Autodesk Inventor part; units mm, degrees
ref_plane "YZ Plane" through (0, 0, 0) normal (1, 0, 0) x (0, 1, 0)
ref_plane "XZ Plane" through (0, 0, 0) normal (0, 1, 0) x (-1, 0, 0)
ref_plane "XY Plane" through (0, 0, 0) normal (0, 0, 1) x (1, 0, 0)
sketch "Sketch1" plane through (0, 0, 0) normal (0, 1, 0) x (-1, 0, 0)
  line L0 (-17.5, 16.9) -> (17.5, 16.9)
  line L1 (17.5, 16.9) -> (17.5, -16.9)
  line L2 (17.5, -16.9) -> (-17.5, -16.9)
  line L3 (-17.5, -16.9) -> (-17.5, 16.9)
  line L4 (-17.5, 16.9) -> (17.5, -16.9) construction
  line L5 (17.5, 16.9) -> (-17.5, -16.9) construction
  point P0 (0, 0)
sketch "Sketch2" plane through (0, 0, 0) normal (0, 1, 0) x (-1, 0, 0)
  line L0 (980.2308, 0) -> (977.7308, 0)
  line L1 (17.4632, -0.049) -> (15.105, -0.049)
  line L2 (12.1095, 2.9465) -> (18.1005, 2.9465)
  line L3 (18.1005, 2.9465) -> (18.1005, -3.0446)
  line L4 (18.1005, -3.0446) -> (12.1095, -3.0446)
  line L5 (12.1095, -3.0446) -> (12.1095, 2.9465)
  line L6 (12.1095, 2.9465) -> (18.1005, -3.0446) construction
  line L7 (18.1005, 2.9465) -> (12.1095, -3.0446) construction
  line L8 (12.4632, 12.2678) -> (18.1005, 12.2678)
  line L9 (18.1005, 12.2678) -> (18.1005, 6.638)
  line L10 (18.1005, 6.638) -> (12.4632, 6.638)
  line L11 (12.4632, 6.638) -> (12.4632, 12.2678)
  line L12 (12.4632, 12.2678) -> (18.1005, 6.638) construction
  line L13 (12.0658, -6.5864) -> (18.1005, -6.5864)
  line L14 (18.1005, -6.5864) -> (18.1005, -12.7382)
  line L15 (18.1005, -12.7382) -> (12.0658, -12.7382)
  line L16 (12.0658, -12.7382) -> (12.0658, -6.5864)
  line L17 (12.0658, -6.5864) -> (18.1005, -12.7382) construction
  line L18 (18.1005, -6.5864) -> (12.0658, -12.7382) construction
  point P0 (0, 0)
  dimension "d2" = 2.5
extrude "Extrusion1" add sketch "Sketch1" along normal blind 4
extrude "Extrusion2" cut sketch "Sketch2" along normal blind 4
fillet "Fillet3" radius 2 1 edges at (17.5, 4, 0)
fillet "Fillet4" radius 2 1 edges at (17.5, 0, 0)
sketch "Sketch3" plane through (0, 4, 0) normal (0, 1, 0) x (1, 0, 0)
  line L0 (-17.5, 3.0446) -> (-12.1095, 3.0446) construction
  line L1 (-12.1095, 3.0446) -> (-12.1095, -2.9465) construction
  line L2 (-12.1095, -2.9465) -> (-17.5, -2.9465) construction
  line L3 (-17.5, -2.9465) -> (-17.5, -6.638) construction
  line L4 (-17.5, -6.638) -> (-12.4632, -6.638) construction
  line L5 (-12.4632, -6.638) -> (-12.4632, -12.2678) construction
  line L6 (-12.4632, -12.2678) -> (-17.5, -12.2678) construction
  line L7 (-17.5, -12.2678) -> (-17.5, -16.9) construction
  line L8 (-17.5, -16.9) -> (15.5, -16.9) construction
  line L9 (15.5, 16.9) -> (-17.5, 16.9) construction
  line L10 (-17.5, 16.9) -> (-17.5, 12.7382) construction
  line L11 (-17.5, 12.7382) -> (-12.0658, 12.7382) construction
  line L12 (-12.0658, 12.7382) -> (-12.0658, 6.5864) construction
  line L13 (-12.0658, 6.5864) -> (-17.5, 6.5864) construction
  line L14 (-17.5, 6.5864) -> (-17.5, 3.0446) construction
  line L15 (-12.1095, 0.049) -> (15.5, 0) construction
  line L16 (-17.5, 16.9) -> (17.5, 16.9) construction
  line L17 (17.5, -16.9) -> (-17.5, -16.9) construction
  line L18 (-9.5803, 7.5215) -> (-9.5803, -7.4785)
  line L19 (-9.5803, -7.4785) -> (3.41, -14.9785)
  line L20 (-9.5803, 7.5215) -> (-7.0803, 6.0781)
  line L21 (-7.0803, 6.0781) -> (-7.0803, -6.0352)
  line L22 (-7.0803, -6.0352) -> (0.91, -10.6484)
  line L23 (0.91, -10.6484) -> (0.91, 1.4648)
  line L24 (0.91, 1.4648) -> (3.41, 0.0215)
  line L25 (3.41, 0.0215) -> (3.41, -14.9785)
  line L26 (15.5, 16.9) -> (15.5, -16.9)
  line L27 (3.41, 16.9) -> (3.41, -16.9) construction
  line L28 (-17.5, -16.9) -> (15.5, -16.9) construction
  line L29 (15.5, 16.9) -> (15.5, 16.9) construction
  line L30 (15.5, 16.9) -> (15.5, -16.9) construction
  line L31 (15.5, -16.9) -> (15.5, -16.9) construction
  line L32 (15.5, -16.9) -> (15.5, 16.9) construction
  dimension "d23" = 2.5
  dimension "d24" = 2.5
  dimension "d25" = 2.5
  dimension "d26" = 15
  dimension "d28" = 15
emboss "Emboss1" sketch "Sketch3" operation cut depth 1 direction (0, -1, 0)
sketch "Sketch4" plane through (0, 4, 0) normal (0, 1, 0) x (1, 0, 0)
  line L0 (-9.5803, 7.5215) -> (-7.0803, 6.0781) construction
  line L1 (-7.0803, 6.0781) -> (-7.0803, -6.0352) construction
  line L2 (-7.0803, -6.0352) -> (0.91, -10.6484) construction
  line L3 (0.91, -10.6484) -> (0.91, 1.4648) construction
  line L4 (0.91, 1.4648) -> (3.41, 0.0215) construction
  line L5 (3.41, 0.0215) -> (3.41, -14.9785) construction
  line L6 (3.41, -14.9785) -> (-9.5803, -7.4785) construction
  line L7 (-9.5803, -7.4785) -> (-9.5803, 7.5215) construction
  line L8 (15.5, 16.9) -> (15.5, -16.9) construction
  line L9 (15.5, 16.9) -> (-17.5, 16.9) construction
  line L10 (-17.5, 16.9) -> (-17.5, 12.7382) construction
  line L11 (-17.5, 12.7382) -> (-12.0658, 12.7382) construction
  line L12 (-12.0658, 12.7382) -> (-12.0658, 6.5864) construction
  line L13 (-12.0658, 6.5864) -> (-17.5, 6.5864) construction
  line L14 (-17.5, 6.5864) -> (-17.5, 3.0446) construction
  line L15 (-17.5, 3.0446) -> (-12.1095, 3.0446) construction
  line L16 (-12.1095, 3.0446) -> (-12.1095, -2.9465) construction
  line L17 (-12.1095, -2.9465) -> (-17.5, -2.9465) construction
  line L18 (-17.5, -2.9465) -> (-17.5, -6.638) construction
  line L19 (-17.5, -6.638) -> (-12.4632, -6.638) construction
  line L20 (-12.4632, -6.638) -> (-12.4632, -12.2678) construction
  line L21 (-12.4632, -12.2678) -> (-17.5, -12.2678) construction
  line L22 (-17.5, -12.2678) -> (-17.5, -16.9) construction
  line L23 (-17.5, -16.9) -> (15.5, -16.9) construction
  line L24 (-12.1095, 0.049) -> (15.5, 0) construction
  line L25 (15.5, -16.9) -> (15.5, 16.9) construction
  line L26 (0.91, 16.9) -> (0.91, -16.9) construction
  line L27 (15.5, -16.9) -> (-17.5, -16.9) construction
  line L28 (0.91, -10.6484) -> (0.91, 1.4648) construction
  line L29 (-7.0803, 6.0781) -> (-7.0803, -6.0352)
  line L30 (-7.0803, -6.0352) -> (0.91, -10.6484)
  line L31 (-7.0803, 6.0781) -> (-7.0803, -6.0352)
  line L32 (-7.0803, -6.0352) -> (0.91, -10.6484)
  line L33 (0.91, -10.6484) -> (0.91, -7.7617)
  line L34 (0.91, -10.6484) -> (0.91, 1.4648)
  line L35 (0.91, -7.7617) -> (-4.5803, -4.5918)
  line L36 (-4.5803, -4.5918) -> (-4.5803, 4.6347)
  line L37 (-4.5803, 4.6347) -> (0.91, 7.8046)
  line L38 (-7.0803, 6.0781) -> (0.91, 10.6913)
  line L39 (0.91, 10.6913) -> (0.91, 7.8046)
  point P0 (0, 0)
  dimension "d29" = 120
  dimension "d30" = 2.5
  dimension "d31" = 2.5
  dimension "d32" = 2.5
emboss "Emboss2" sketch "Sketch4" operation cut depth 1.5 direction (0, -1, 0)
sketch "Sketch5" plane through (0, 4, 0) normal (0, 1, 0) x (1, 0, 0)
  line L0 (-4.5803, -4.5918) -> (0.91, -7.7617) construction
  line L1 (0.91, -7.7617) -> (0.91, 1.4648) construction
  line L2 (0.91, 1.4648) -> (3.41, 0.0215) construction
  line L3 (3.41, 0.0215) -> (3.41, -14.9785) construction
  line L4 (3.41, -14.9785) -> (-9.5803, -7.4785) construction
  line L5 (-9.5803, -7.4785) -> (-9.5803, 7.5215) construction
  line L6 (-9.5803, 7.5215) -> (-7.0803, 6.0781) construction
  line L7 (-7.0803, 6.0781) -> (0.91, 10.6913) construction
  line L8 (0.91, 10.6913) -> (0.91, 7.8046) construction
  line L9 (0.91, 7.8046) -> (-4.5803, 4.6347) construction
  line L10 (-4.5803, 4.6347) -> (-4.5803, -4.5918) construction
  line L11 (15.5, 16.9) -> (15.5, -16.9) construction
  line L12 (15.5, 16.9) -> (-17.5, 16.9) construction
  line L13 (-17.5, 16.9) -> (-17.5, 12.7382) construction
  line L14 (-17.5, 12.7382) -> (-12.0658, 12.7382) construction
  line L15 (-12.0658, 12.7382) -> (-12.0658, 6.5864) construction
  line L16 (-12.0658, 6.5864) -> (-17.5, 6.5864) construction
  line L17 (-17.5, 6.5864) -> (-17.5, 3.0446) construction
  line L18 (-17.5, 3.0446) -> (-12.1095, 3.0446) construction
  line L19 (-12.1095, 3.0446) -> (-12.1095, -2.9465) construction
  line L20 (-12.1095, -2.9465) -> (-17.5, -2.9465) construction
  line L21 (-17.5, -2.9465) -> (-17.5, -6.638) construction
  line L22 (-17.5, -6.638) -> (-12.4632, -6.638) construction
  line L23 (-12.4632, -6.638) -> (-12.4632, -12.2678) construction
  line L24 (-12.4632, -12.2678) -> (-17.5, -12.2678) construction
  line L25 (-17.5, -12.2678) -> (-17.5, -16.9) construction
  line L26 (-17.5, -16.9) -> (15.5, -16.9) construction
  line L27 (-7.0803, 6.0781) -> (0.91, 10.6913)
  line L28 (-9.5803, 7.5215) -> (-7.0803, 6.0781)
  line L29 (-7.0803, 6.0781) -> (0.91, 10.6913)
  line L30 (0.91, 10.6913) -> (0.91, 7.8046)
  line L31 (0.91, 10.6913) -> (0.91, 7.8046)
  line L32 (0.91, 16.9) -> (0.91, -16.9) construction
  line L33 (0.91, -7.7617) -> (0.91, 1.4648) construction
  line L34 (-9.5803, 7.5215) -> (0.91, 13.5781)
  line L35 (0.91, 13.5781) -> (13.9004, 6.0781)
  line L36 (13.9004, 6.0781) -> (13.9004, 3.1913)
  line L37 (13.9004, 3.1913) -> (5.91, -1.4219)
  line L38 (5.91, -1.4219) -> (5.91, -7.6363)
  line L39 (5.91, -7.6363) -> (11.2919, -4.5291)
  line L40 (13.9004, -6.0352) -> (13.9004, -8.9219)
  line L41 (3.41, -14.9785) -> (-9.5803, -7.4785)
  line L42 (13.9004, -8.9219) -> (3.41, -14.9785)
  line L43 (0.91, 1.4648) -> (3.41, 0.0215)
  line L44 (3.41, -14.9785) -> (3.41, 0.0215)
  line L45 (3.41, 0.0215) -> (0.91, 1.4648)
  line L46 (0.91, 7.8046) -> (-4.5803, 4.6347)
  line L47 (0.91, 7.8046) -> (0.91, 10.6913)
  line L48 (3.41, 0.0215) -> (3.41, -14.9785)
  line L49 (0.91, 1.4648) -> (6.4004, 4.6347)
  line L50 (6.4004, 4.6347) -> (0.91, 7.8046)
  line L51 (13.9004, -6.0352) -> (11.2919, -4.5291)
  line L52 (-7.1521, -6.1594) -> (3.41, -12.0918) construction
  line L53 (-4.5803, -4.5918) -> (0.91, -7.7617) construction
  line L54 (-4.5803, -4.5918) -> (3.41, -9.0797) construction
  line L55 (3.41, -9.0797) -> (14.5341, -2.6572) construction
  line L56 (3.41, 0.0215) -> (13.9004, 6.0781) construction
  line L57 (3.41, -12.0918) -> (19.1495, -3.0046) construction
  line L58 (6.4004, 4.6347) -> (9.227, 5.8895) construction
  line L59 (0.91, 10.6913) -> (0.91, 7.8046) construction
  line L60 (9.227, 5.8895) -> (0.91, 10.6913) construction
  point P0 (0, 0)
  dimension "d35" = 60
  dimension "d36" = 2.5
  dimension "d39" = 120
  dimension "d42" = 120
  dimension "d43" = 2.5
emboss "Emboss3" sketch "Sketch5" operation cut depth 2 direction (0, -1, 0)
equation "\"d24\" = d23"
equation "\"d25\" = d23"
equation "\"d28\" = d26"
equation "\"d30\" = d23"
equation "\"d31\" = d23"
equation "\"d32\" = d23"
equation "\"d36\" = d23"
equation "\"d43\" = d23"
properties part number "schablone"
Check sheet for the modelled part. Datum: model origin and axes. Units: mm. A direction names the side the tool comes from. Coordinates: 2 decimals unless noted, no trailing zeros. Order: outer loops, then holes, each group sorted by start corner. A loop starts at its lowest first (then second) coordinate and runs counter-clockwise, first axis right, second up. Notation, with made-up numbers: (-35.75, -2.5) -> (12.25, -2.5) arc R27 cw to (12.25, 25.5) -> close; hole circle Ø7 at (30, -28). An arc over 180 degrees is marked (long way). Write each question's results on one line, items separated by ' | '. Start each with the question number.
1) Section check A-A (y = 3.6). Count the separate pieces of the cut face and the enclosed holes in it, and give its area (3 significant figures).
2) Draft check along X on faces 4 (the face through (-12.066, 2, -10)), 5 (the face through (-15, 2, 6.638)), 6 (the face through (5.91, 3, 5)), 7 (the face through (16.9, 0.57, 0.24)). Enter one of: pulls with the +X half, pulls with the -X half, needs draft (parallel to the pull), parting line crosses it, or undercut.
3) Section check C-C (x = 7). Enter the section's corners in (y, z), and give its area (3 significant figures).
4) Depth check by flat-ended pin: pin 1 (1.2 mm diameter, centred on y = 2, z = -1, fed in from -X); pin 2 (0.8 mm diameter, centred on y = 2.5, z = 7, fed in from +X). Enter the tip coordinate at first touch or a pass-through.
5) Section check B-B (x = -14). Enter the section's corners in (y, z).
6) Material ranges on line 1 along Z through (x, y) = (-13.5, 1.5); line 2 along X through (y, z) = (2.1, 1.5); line 3 along X through (y, z) = (3.35, 1.5), recorded low to high.
7) Set-up check for faces 1 (the face through (-15, 2, -12.738)), 2 (the face through (9.849, 3.014, -0.852)), 3 (the face through (-17.5, 2, 5)): record each of +Z, -Z, +X, -X, +Y, -Y from which the full face is reachable in a straight line by a thin tool's end or side.
8) Section check D-D (y = 1.35). Enter the section's corners in (x, z).
Checked values:
1) separate pieces: 2 | enclosed holes: 1 | area: 691 mm²
2) face 4: pulls with the -X half | face 5: needs draft | face 6: undercut | face 7: pulls with the +X half
3) outline: (0, -16.9) -> (4, -16.9) -> (4, -10.06) -> (2, -10.06) -> (2, 0.79) -> (4, 0.79) -> (4, 7.01) -> (2, 7.01) -> (2, 12.91) -> (4, 12.91) -> (4, 16.9) -> (0, 16.9) -> close | area: 102 mm²
4) pin 1: x = -12.11 | pin 2: x = 17.5
5) outline: (0, -16.9) -> (4, -16.9) -> (4, -12.74) -> (0, -12.74) -> close; (0, -6.59) -> (4, -6.59) -> (4, -3.04) -> (0, -3.04) -> close; (0, 2.95) -> (4, 2.95) -> (4, 6.64) -> (0, 6.64) -> close; (0, 12.27) -> (4, 12.27) -> (4, 16.9) -> (0, 16.9) -> close
6) line 1: -16.9 to -12.74, -6.59 to -3.04, 2.95 to 6.64, 12.27 to 16.9 | line 2: -12.11 to 3.41, 5.91 to 17.5 | line 3: -12.11 to -9.58, -4.58 to 0.91, 5.91 to 16.98
7) face 1: -X, +Y, -Y | face 2: +Y | face 3: +Z, -Z, -X, +Y, -Y
8) outline: (-17.5, -16.9) -> (17.39, -16.9) -> (17.39, 16.9) -> (-17.5, 16.9) -> (-17.5, 12.27) -> (-12.46, 12.27) -> (-12.46, 6.64) -> (-17.5, 6.64) -> (-17.5, 2.95) -> (-12.11, 2.95) -> (-12.11, -3.04) -> (-17.5, -3.04) -> (-17.5, -6.59) -> (-12.07, -6.59) -> (-12.07, -12.74) -> (-17.5, -12.74) -> close
